```python
from build123d import *

# Parameters (mm, degrees)
F0_W     = 3
F0_H     = 10
F1_DEPTH = 3.5
F2_W     = 1
F2_H     = 3
F3_DEPTH = 25
F4_DEPTH = 2.1
F5_START = -11
F5_DEPTH = 4


with BuildPart() as f1:
    # F0 (on Front) → F1 (new body, symmetric)
    with BuildSketch(Plane.XZ):
        with Locations((-5.06, 5)):
            Rectangle(F0_W, F0_H)
        Polygon((-3.56, 0), (-6.56, 0), (-6.56, -3), (6.44, -3), (6.44, 0), (3.44, 0), align=None)
        with Locations((4.94, 5)):
            Rectangle(F0_W, F0_H)
    extrude(amount=F1_DEPTH, both=True)

    # F2 (on face) → F3 (cut, symmetric)
    with BuildSketch(Plane(origin=(-6.56, 0, 0), x_dir=(0, -1, 0), z_dir=(-1, 0, 0))):
        with Locations((0, 6)):
            Rectangle(F2_W, F2_H)
    extrude(amount=F3_DEPTH, both=True, mode=Mode.SUBTRACT)

    # F2 (on face) → F4 (cut)
    with BuildSketch(Plane(origin=(-6.56, 0, 0), x_dir=(0, -1, 0), z_dir=(-1, 0, 0))):
        with BuildLine():
            Line((-0.5, 7.5), (-0.5, 8.6024027359))
            ThreePointArc((-0.5, 8.6024027359), (-2.65, 6), (-0.5, 3.3975972641))
            Line((-0.5, 3.3975972641), (-0.5, 4.5))
            Line((-0.5, 4.5), (-0.5, 7.5))
        make_face()
        with BuildLine():
            ThreePointArc((0.5, 3.3975972641), (2.0429757708, 4.312175957), (2.65, 6))
            ThreePointArc((2.65, 6), (2.0429757708, 7.687824043), (0.5, 8.6024027359))
            Line((0.5, 8.6024027359), (0.5, 7.5))
            Line((0.5, 7.5), (0.5, 4.5))
            Line((0.5, 4.5), (0.5, 3.3975972641))
        make_face()
        with BuildLine():
            Line((0.5, 7.5), (0.5, 8.6024027359))
            ThreePointArc((0.5, 8.6024027359), (0, 8.65), (-0.5, 8.6024027359))
            Line((-0.5, 8.6024027359), (-0.5, 7.5))
            Line((-0.5, 7.5), (0.5, 7.5))
        make_face()
        with BuildLine():
            ThreePointArc((-0.5, 3.3975972641), (0, 3.35), (0.5, 3.3975972641))
            Line((0.5, 3.3975972641), (0.5, 4.5))
            Line((0.5, 4.5), (-0.5, 4.5))
            Line((-0.5, 4.5), (-0.5, 3.3975972641))
        make_face()
    extrude(amount=-F4_DEPTH, mode=Mode.SUBTRACT)

    # F2 (on face) → F5 (cut)
    with BuildSketch(Plane(origin=(-6.56, 0, 0), x_dir=(0, -1, 0), z_dir=(-1, 0, 0)).offset(F5_START)):
        with BuildLine():
            Line((-0.5, 7.5), (-0.5, 8.6024027359))
            ThreePointArc((-0.5, 8.6024027359), (-2.65, 6), (-0.5, 3.3975972641))
            Line((-0.5, 3.3975972641), (-0.5, 4.5))
            Line((-0.5, 4.5), (-0.5, 7.5))
        make_face()
        with BuildLine():
            Line((0.5, 7.5), (0.5, 8.6024027359))
            ThreePointArc((0.5, 8.6024027359), (0, 8.65), (-0.5, 8.6024027359))
            Line((-0.5, 8.6024027359), (-0.5, 7.5))
            Line((-0.5, 7.5), (0.5, 7.5))
        make_face()
        with BuildLine():
            ThreePointArc((-0.5, 3.3975972641), (0, 3.35), (0.5, 3.3975972641))
            Line((0.5, 3.3975972641), (0.5, 4.5))
            Line((0.5, 4.5), (-0.5, 4.5))
            Line((-0.5, 4.5), (-0.5, 3.3975972641))
        make_face()
        with BuildLine():
            ThreePointArc((0.5, 3.3975972641), (2.0429757708, 4.312175957), (2.65, 6))
            ThreePointArc((2.65, 6), (2.0429757708, 7.687824043), (0.5, 8.6024027359))
            Line((0.5, 8.6024027359), (0.5, 7.5))
            Line((0.5, 7.5), (0.5, 4.5))
            Line((0.5, 4.5), (0.5, 3.3975972641))
        make_face()
    extrude(amount=-F5_DEPTH, mode=Mode.SUBTRACT)


solid = f1.part
```
The model under review builds one solid part; all positions refer to its coordinate system, in mm. A direction names the side the tool comes from. Round coordinates to 2 decimals unless told otherwise and drop trailing zeros. Loops run counter-clockwise (first coordinate to the right, second up) from the corner with the lowest first, then second, coordinate; pieces in that order, holes last. Notation, with made-up numbers: (18.5, 22.25) - (62.5, 22.25) arc R33 ccw to (62.5, 51.25) - close; hole circle Ø7 at (-25, 12.5). An arc over 180 degrees is marked (long way). Write each question's results on one line, items separated by ' | '. Start each with the question number.
Q1. Tool access review of faces 1 (the flat face through (-4.46, -1, 6)), 2 (the flat face through (4.44, -1, 6)), 3 (the flat face through (-4, 0, 4.5)), 4 (the flat face through (3.44, -1, 5)): name each direction out of +Z, -Z, +X, -X, +Y, -Y from which nothing blocks a thin tool from reaching the whole face with its end or side.
Q2. Draft analysis for pull direction Z (two halves, no side actions). For faces 5 (the flat face through (-5, 0, 10)), 6 (the flat face through (6.44, 0, 2)), 7 (the flat face through (4, -0.5, 6)), state which applies: pulls with the +Z half, pulls with the -Z half, needs draft (parallel to the pull), parting line crosses it, or undercut.
Q3. Wall thickness on line 1 along X through (y, z) = (1.75, 3); line 2 along X through (y, z) = (-2.25, 5); line 3 along Z through (x, y) = (-2.25, -3): over which ranges is each line inside the solid? List them lowest first. Write a range as [from, to].
Q4. Take a section at D-D on y = 0.75. Give the boundary of the cut face in (x, z).
Q5. Insertion check: P1, Ø4, axis at x = -1, y = 0, coming from the +Z side; P2, Ø1.6, axis at y = -0.5, z = 6, coming from the +X side. Each pin has a flat end and moves straight along its axis. Give the tip position at first contact, or say it passes through.
Q6. Take a section at B-B on x = -4.75. Give the boundary of the cut face in (y, z).
Q7. Take a section at C-C on z = 5.5. Give the boundary of the cut face in (x, y), plus the area to 3 significant figures.
Q8. Take a section at A-A on z = 2. Give the boundary of the cut face in (x, y), plus the area to 3 significant figures.
Data:
1) face 1: -X | face 2: +X | face 3: +X, -X | face 4: +Z, +Y, -Y
2) face 5: pulls with the +Z half | face 6: needs draft | face 7: undercut
3) line 1: x = [-6.56, -3.56], [3.44, 6.44] | line 2: x = [-4.46, -3.56], [3.44, 4.44] | line 3: z = [-3, 0]
4) outline: (-6.56, -3) - (6.44, -3) - (6.44, 3.46) - (4.44, 3.46) - (4.44, 8.54) - (6.44, 8.54) - (6.44, 10) - (3.44, 10) - (3.44, 0) - (-3.56, 0) - (-3.56, 10) - (-6.56, 10) - (-6.56, 8.54) - (-4.46, 8.54) - (-4.46, 3.46) - (-6.56, 3.46) - close
5) P1: stops at z = 0 | P2: stops at x = 4.44
6) outline: (-3.5, -3) - (3.5, -3) - (3.5, 10) - (-3.5, 10) - close; hole circle Ø5.3 at (0, 6)
7) outline: (-6.56, -3.5) - (-3.56, -3.5) - (-3.56, -0.5) - (-4.46, -0.5) - (-4.46, -2.6) - (-6.56, -2.6) - close; (-6.56, 2.6) - (-4.46, 2.6) - (-4.46, 0.5) - (-3.56, 0.5) - (-3.56, 3.5) - (-6.56, 3.5) - close; (3.44, -3.5) - (6.44, -3.5) - (6.44, -2.6) - (4.44, -2.6) - (4.44, -0.5) - (3.44, -0.5) - close; (3.44, 0.5) - (4.44, 0.5) - (4.44, 2.6) - (6.44, 2.6) - (6.44, 3.5) - (3.44, 3.5) - close | area: 18.8 mm²
8) outline: (-6.56, -3.5) - (-3.56, -3.5) - (-3.56, 3.5) - (-6.56, 3.5) - close; (3.44, -3.5) - (6.44, -3.5) - (6.44, 3.5) - (3.44, 3.5) - close | area: 42.0 mm²
